Autodesk Fusion 360 part; units mm, degrees
sketch "Sketch1" plane through (0, 0, 0) normal (0, 0, 1) x (1, 0, 0)
  circle A0 centre (0, 0) radius 3.7
  circle A1 centre (0, 0) radius 6
  line L0 (-25, -13.2) -> (25, -13.2)
  line L1 (25, -13.2) -> (25, -17.2)
  line L2 (25, -17.2) -> (-25, -17.2)
  line L3 (-25, -17.2) -> (-25, -13.2)
  line L4 (-6, 0) -> (6, 0)
  line L5 (6, 0) -> (6, -13.2)
  line L6 (6, -13.2) -> (-6, -13.2)
  line L7 (-6, -13.2) -> (-6, 0)
  point P0 (0, -13.2)
  dimension "d1" = 7.4
  dimension "d2" = 12
  dimension "d7" = 50
  dimension "d8" = 13.2
  dimension "d30" = 4
extrude "Extrude1" add sketch "Sketch1" along normal blind 2 contours A0 L4 | A0 A1 L4 | A0 A1 L4 | A0 L4
extrude "Extrude2" add sketch "Sketch1" along normal blind 18 contours A0 A1 L4 | A0 A1 L4
extrude "Extrude3" add sketch "Sketch1" along normal blind 12 contours A1 L0 L5 L6 L7
extrude "Extrude9" add 1 faces at (2, -13.2, 8) along direction (0, -1, 0) blind 1
draft "Draft1" angle 35 neutral plane through (-6, -13.2, 0) pull (0, 0, -1) 1 faces at (2, -14.2, 8)
sketch "Sketch5" plane through (0, -9.5283, -6.6718) normal (0, -0.8192, -0.5736) x (1, 0, 0)
  line L0 (-6, 8.1448) -> (6, 8.1448)
  line L1 (6, 8.1448) -> (6, 22.7941)
  line L2 (6, 22.7941) -> (-6, 22.7941)
  line L3 (-6, 22.7941) -> (-6, 8.1448)
  circle A0 centre (0, 22.2702) radius 35
  dimension "d44" = 70
extrude "Extrude10" add sketch "Sketch5" along direction (0, -0.906308, -0.422618) blind 1.2 contours L0 L1 L2 L3 | A0
Can you work these out from the model? Positions are in its coordinate system, mm. A direction names the side the tool comes from. Round coordinates to 2 decimals unless told otherwise and drop trailing zeros. Use a Markdown table: item, result.
Item 1: If I drill on line 1 along Y through (x, z) = (0, 13.25); line 2 along X through (y, z) = (0, 11); line 3 along Y through (x, z) = (0, 13.75), over which ranges is the centre line in solid material (lowest first)? Write a range as [from, to].
Found:
| item | result |
|---|---|
| line 1 | y = [-24.92, -23.48], [-6, -3.7], [3.7, 6] |
| line 2 | x = [-6, -3.7], [3.7, 6] |
| line 3 | y = [-25.27, -23.83], [-6, -3.7], [3.7, 6] |
Item 2: For pin 1 Ø8 at (x, z) = (26.5, 18.5) entering from +Y; pin 2 Ø8 at (x, y) = (24, -20) entering from +Z; pin 3 Ø3.5 at (x, y) = (0.5, -8) entering from -Z, each with a flat end and sliding along its axis, tell me the tip position at first contact or that it passes through.
Found:
| item | result |
|---|---|
| pin 1 | stops at y = -24.35 |
| pin 2 | stops at z = 14 |
| pin 3 | stops at z = -13.41 |
Item 3: We'd pull the mould along Z, two halves only. Please class faces 1 (the face through (0, -4, 0)), 2 (the face through (-1.301, 5.857, 10.874)), 3 (the face through (0, -14, 12)): released by +Z, released by -Z, zero draft, split by the parting line, or undercut.
Found:
| item | result |
|---|---|
| face 1 | undercut |
| face 2 | zero draft |
| face 3 | released by +Z |
Item 4: Which directions (+Z, -Z, +X, -X, +Y, -Y) give clear straight access to the entire face, cutting with the end or side of a thin tool? Please do faces 4 (the face through (-6, -9, 6)), 5 (the face through (-0.802, 3.612, 9.888)), 6 (the face through (-0.49, -23.671, 11.465)), 7 (the face through (6, -9, 6)), 8 (the face through (-3, -3, 18)).
Found:
| item | result |
|---|---|
| face 4 | +Z, -X, +Y |
| face 5 | +Z |
| face 6 | -Z, +X, -X, -Y |
| face 7 | +Z, +X, +Y |
| face 8 | +Z, +X, -X, +Y |
Item 5: I want a section at A-A (z = 13). State how many separate pieces and enclosed holes the cut face has, and give its area (3 significant figures).
Found:
| item | result |
|---|---|
| separate pieces | 2 |
| enclosed holes | 1 |
| area | 171 mm2 |
